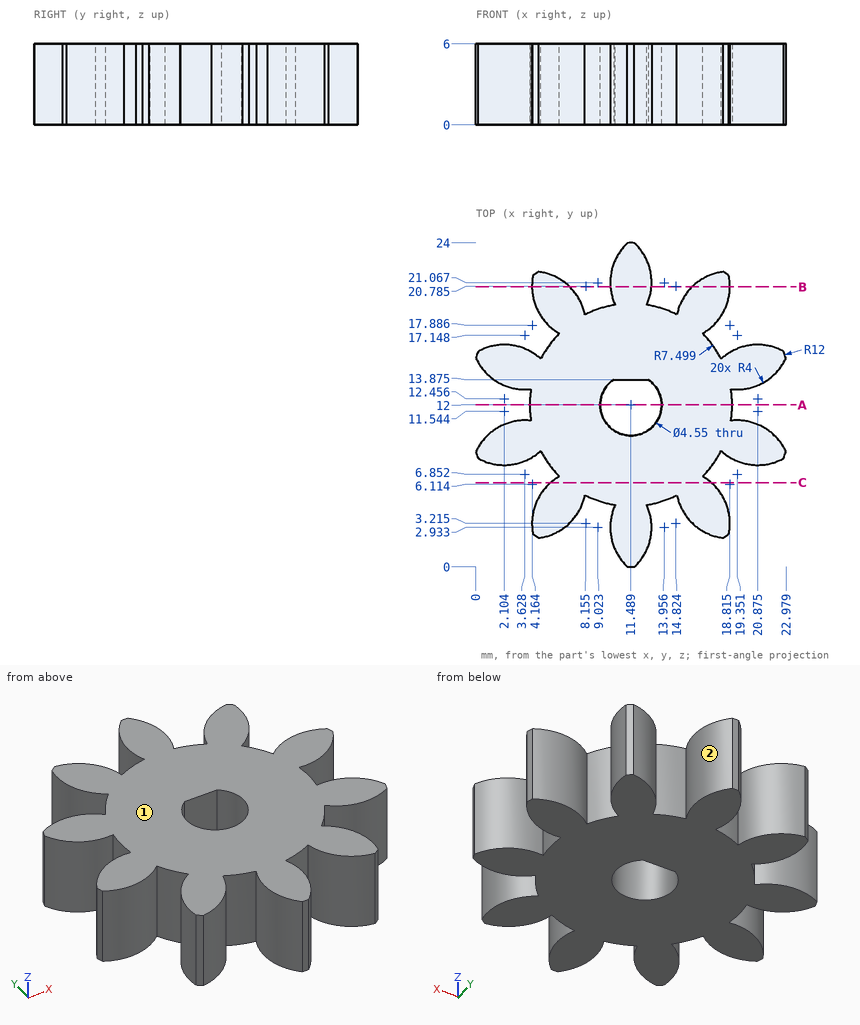
Design review of the part shown in the three views and the two pictorial views. Dimensions are in mm from the part's minimum x, y and z. Give positions to 0.01 mm unless a question says otherwise; leave off trailing zeros. Loops run counter-clockwise (first coordinate to the right, second up) from the corner with the lowest first, then second, coordinate; pieces in that order, holes last. Notation, with made-up numbers: (-16.5, 17.5) -> (38.5, 17.5) arc R17 ccw to (38.5, 39.5) -> close; hole circle Ø6 at (5, 61.5). An arc over 180 degrees is marked (long way). Put each result on its own line as item: value. Start each with the question number.
1. We need section A-A on y = 12. State the section outline as (x, z) points (1 decimal).
2. We need section B-B on y = 20.75. State the section outline as (x, z) points (1 decimal).
3. We need section C-C on y = 6.25. State the section outline as (x, z) points.
4. Wall thickness on probe 1 along X at (y, z) = (4, 0.5) (1 decimal); probe 2 along X at (y, z) = (12, 4.2) (1 decimal); probe 3 along Y at (x, z) = (5.5, 0.35) (1 decimal): over which ranges is each line inside the solid? List them lowest first.
5. Clearance check with a flat-ended pin moving along its axis: P1, Ø2.5, axis at x = 11.49, y = 12, coming from the +Z side. State where the tip first meets the part, or that it passes through.
6. Mouldability with a two-part tool opening along X and no side actions: class the marked faces 1 and 2 as released by +X, released by -X, zero draft, split by the parting line, or undercut.
Determined:
1. outline: (4, 0) -> (9.2, 0) -> (9.2, 6) -> (4, 6) -> close; (13.8, 0) -> (19, 0) -> (19, 6) -> (13.8, 6) -> close
2. outline: (4.2, 0) -> (7, 0) -> (7, 6) -> (4.2, 6) -> close; (10, 0) -> (13, 0) -> (13, 6) -> (10, 6) -> close; (16, 0) -> (18.8, 0) -> (18.8, 6) -> (16, 6) -> close
3. outline: (5.55, 0) -> (17.43, 0) -> (17.43, 6) -> (5.55, 6) -> close
4. probe 1: 4.2 to 7.6, 10.1 to 12.9, 15.4 to 18.7
4. probe 2: 4 to 9.2, 13.8 to 19
4. probe 3: 2.3 to 6.2, 7.5 to 16.5, 17.8 to 21.7
5. P1: through
6. face 1: zero draft
6. face 2: undercut
